```python
from build123d import *

# Parameters (mm, degrees)
F0_R     = 2.5
F1_DEPTH = 114.3
F2_D     = 4.2
F2_DEPTH = 20
F2_TIP   = 1.2618073


with BuildPart() as f1:
    # F0 (on Top) → F1 (new body)
    with BuildSketch(Plane.XY):
        Polygon((23.8125, 14.2875), (11.90625, 14.2875), (0, 14.2875), (0, 0), (11.90625, 0), (23.8125, 0), align=None)
        with Locations((5.953125, 7.14375)):
            Circle(F0_R, mode=Mode.SUBTRACT)
        with Locations((17.859375, 7.14375)):
            Circle(F0_R, mode=Mode.SUBTRACT)
        with Locations((5.953125, 7.14375)):
            Circle(F0_R)
        with Locations((17.859375, 7.14375)):
            Circle(F0_R)
    extrude(amount=F1_DEPTH)

    # F2
    with Locations(Plane(origin=(0, 0, 0), x_dir=(1, 0, 0), z_dir=(0, 0, -1))):
        with Locations((17.859375, -7.14375), (5.953125, -7.14375)):
            Hole(F2_D / 2, depth=F2_DEPTH)
            with Locations((0, 0, -(F2_DEPTH + F2_TIP / 2))):  # 118° drill point
                Cone(0, F2_D / 2, F2_TIP, mode=Mode.SUBTRACT)


solid = f1.part
```
Work out the finished part from the listing and answer in its coordinate system (mm). A direction names the side the tool comes from. Coordinates: 2 decimals unless noted, no trailing zeros. Answer as CSV lines item,"result".
Q1. A tool of negligible diameter and unlimited length cuts with its end or side. For faces 1 (the face through (23.812, 7, 56)), 2 (the face through (15.9, 7.9, 10.1)), from which of +Z, -Z, +X, -X, +Y, -Y can it reach the whole face along a straight path? Write none if from no direction.
Findings:
face 1,"+Z, -Z, +X, +Y, -Y"
face 2,"-Z"
Q2. This flat-tipped pin is pushed along its axis until it touches: pin 1 (6 mm diameter, centred on y = 9.5, z = 99.5, fed in from -X). Where does it stop, or does it pass through?
Findings:
pin 1,"stops at x = 0"
Q3. Find the intervals of material crossed by probe 1 along Y at (x, z) = (17, 14.5), in increasing order.
Findings:
probe 1,"y = 0 to 5.23, 9.06 to 14.29"
Q4. For a pull along Y with two mould halves and no side action, classify faces 3 (the face through (4.984, 9.007, 10.14)), 4 (the face through (12, 0, 56)), 5 (the face through (12, 7, 114.3)), 6 (the face through (12, 14.288, 56)) as +Y half, -Y half, draft (parallel to the pull), parting line (faces both ways), or undercut.
Findings:
face 3,"undercut"
face 4,"-Y half"
face 5,"draft"
face 6,"+Y half"
